from build123d import *

# Parameters (mm, degrees)
F0_W      = 31
F0_H      = 41
F1_DEPTH  = 12
F2_T      = -2
F3_R      = 1.5
F4_DEPTH  = 25
F6_DEPTH  = 25
F7_W      = 14.291796
F7_H      = 4
F8_DEPTH  = 1
F9_W      = 12
F9_H      = 2
F10_DEPTH = 11
F11_W     = 23
F11_H     = 30
F12_DEPTH = 12
F13_W     = 19
F13_H     = 28
F14_DEPTH = 7
F15_W     = 19
F15_H     = 4
F16_DEPTH = 4
F18_DEPTH = 25
F19_R     = 3.5
F20_DEPTH = 25
F21_W     = 27
F21_H     = 27
F22_DEPTH = 12
F23_W     = 27
F23_H     = 27
F23_W_2   = 15
F23_H_2   = 15
F24_DEPTH = 1
F25_W     = 10.156876
F25_H     = 2
F26_DEPTH = 10
F27_W     = 10
F27_H     = 2
F28_DEPTH = 7


with BuildPart() as f1:
    # F0 (on Top) → F1 (new body)
    with BuildSketch(Plane.XY):
        with Locations((15.5, 20.5)):
            Rectangle(F0_W, F0_H)
    extrude(amount=F1_DEPTH)

    # F2
    f2_openings = [f1.faces().sort_by_distance(p)[0] for p in [
        (15.5, 20.5, 12),
    ]]
    offset(amount=F2_T, openings=f2_openings)

    # F3 (on face) → F4 (cut)
    with BuildSketch(Plane.XY.offset(2)):
        with Locations((5, 36)):
            Circle(F3_R)
        with Locations((26, 36)):
            Circle(F3_R)
        with Locations((26, 5)):
            Circle(F3_R)
        with Locations((5, 5)):
            Circle(F3_R)
    extrude(amount=-F4_DEPTH, mode=Mode.SUBTRACT)

    # F5 (on face) → F6 (cut)
    with BuildSketch(Plane.XY.offset(2)):
        with BuildLine():
            ThreePointArc((25, 32.645898), (23.525126, 33.525126), (22.645898, 35))
            Line((22.645898, 35), (8.354102, 35))
            ThreePointArc((8.354102, 35), (7.474874, 33.525126), (6, 32.645898))
            Line((6, 32.645898), (6, 8.354102))
            ThreePointArc((6, 8.354102), (7.474874, 7.474874), (8.354102, 6))
            Line((8.354102, 6), (22.645898, 6))
            ThreePointArc((22.645898, 6), (23.525126, 7.474874), (25, 8.354102))
            Line((25, 8.354102), (25, 32.645898))
        make_face()
    extrude(amount=-F6_DEPTH, mode=Mode.SUBTRACT)

    # F7 (on face) → F8 (cut)
    with BuildSketch(Plane.XY.offset(2)):
        with Locations((15.5, 4)):
            Rectangle(F7_W, F7_H)
    extrude(amount=-F8_DEPTH, mode=Mode.SUBTRACT)

    # F9 (on face) → F10 (cut)
    with BuildSketch(Plane.XY.offset(12)):
        with Locations((15.5, 1)):
            Rectangle(F9_W, F9_H)
    extrude(amount=-F10_DEPTH, mode=Mode.SUBTRACT)

    # F11 (on face) → F12 (join)
    with BuildSketch(Plane(origin=(0, 0, 0), x_dir=(1, 0, 0), z_dir=(0, 0, -1))):
        with Locations((15.5, 15)):
            Rectangle(F11_W, F11_H)
    extrude(amount=-F12_DEPTH)

    # F13 (on face) → F14 (cut)
    with BuildSketch(Plane.XY.offset(12)):
        with Locations((15.5, -14)):
            Rectangle(F13_W, F13_H)
    extrude(amount=-F14_DEPTH, mode=Mode.SUBTRACT)

    # F15 (on face) → F16 (cut)
    with BuildSketch(Plane.XY.offset(5)):
        with Locations((15.5, -2)):
            Rectangle(F15_W, F15_H)
    extrude(amount=-F16_DEPTH, mode=Mode.SUBTRACT)

    # F17 (on face) → F18 (cut)
    with BuildSketch(Plane.XY.offset(5)):
        Polygon((25, -4), (21, -4), (10, -4), (10, -24), (21, -24), (21, -20), (25, -20), align=None)
    extrude(amount=-F18_DEPTH, mode=Mode.SUBTRACT)

    # F19 (on face) → F20 (cut)
    with BuildSketch(Plane.XZ.offset(-39)):
        with Locations((13.913386, 6.684771)):
            Circle(F19_R)
    extrude(amount=-F20_DEPTH, mode=Mode.SUBTRACT)

    # F21 (on face) → F22 (join)
    with BuildSketch(Plane.XY.offset(12)):
        Polygon((29, 41), (31, 41), (31, 113), (0, 113), (0, 41), (2, 41), (2, 82), (29, 82), align=None)
        with Locations((15.5, 97.5)):
            Rectangle(F21_W, F21_H, mode=Mode.SUBTRACT)
    extrude(amount=-F22_DEPTH)

    # F23 (on face) → F24 (join)
    with BuildSketch(Plane(origin=(0, 0, 0), x_dir=(1, 0, 0), z_dir=(0, 0, -1))):
        with Locations((15.5, -97.5)):
            Rectangle(F23_W, F23_H)
        with Locations((15.5, -97.5)):
            Rectangle(F23_W_2, F23_H_2, mode=Mode.SUBTRACT)
    extrude(amount=-F24_DEPTH)

    # F25 (on face) → F26 (cut)
    with BuildSketch(Plane.XY.offset(12)):
        with Locations((15.545943, 83)):
            Rectangle(F25_W, F25_H)
    extrude(amount=-F26_DEPTH, mode=Mode.SUBTRACT)

    # F27 (on face) → F28 (cut)
    with BuildSketch(Plane.XY.offset(12)):
        with Locations((15.5, -29)):
            Rectangle(F27_W, F27_H)
    extrude(amount=-F28_DEPTH, mode=Mode.SUBTRACT)


solid = f1.part
Source: CAD feature listing. Evaluate the final solid. Frame: model axes, mm. A direction names the side the tool comes from. Give positions to 0.01 mm unless a question says otherwise; leave off trailing zeros. Order: outer loops, then holes, each group sorted by start corner. A loop starts at its lowest first (then second) coordinate and runs counter-clockwise, first axis right, second up. Notation, with made-up numbers: (25.5, 78) -> (80.5, 78) arc R17 ccw to (80.5, 97) -> close; hole circle Ø7 at (67, 53.5). An arc over 180 degrees is marked (long way). Use a Markdown table: item, result.
1) Mould query, pull axis Y, two halves, no side actions, for faces 4 (the flat face through (15.3, -30, 4.6)), 5 (the cylindrical face through (6.386, 4.425, 1.014)), 6 (the flat face through (0, 57, 6)). Classes: +Y half, -Y half, draft (parallel to the pull), parting line (faces both ways), or undercut.
Answer list:
| item | result |
|---|---|
| face 4 | -Y half |
| face 5 | undercut |
| face 6 | draft |
2) Section query B-B, the plane y = 62. Return the cut outline in (x, z).
Answer list:
| item | result |
|---|---|
| outline | (0, 0) -> (2, 0) -> (2, 12) -> (0, 12) -> close; (29, 0) -> (31, 0) -> (31, 12) -> (29, 12) -> close |
3) Section query C-C, the plane y = 17. Return the cut outline in (x, z), then the cut area to 3 significant figures.
Answer list:
| item | result |
|---|---|
| outline | (0, 0) -> (6, 0) -> (6, 2) -> (2, 2) -> (2, 12) -> (0, 12) -> close; (25, 0) -> (31, 0) -> (31, 12) -> (29, 12) -> (29, 2) -> (25, 2) -> close |
| area | 64.0 mm² |
4) Contact query for flat-ended pins moving along their axis: P1, Ø4, axis at x = 5, y = 5, coming from the +Z side; P2, Ø2.5, axis at x = 26, y = 36, coming from the +Z side. Output: stop coordinate, or through.
Answer list:
| item | result |
|---|---|
| P1 | z = 2 |
| P2 | through |
5) Ray query, line 1 along Y through (x, z) = (5, 0.9); line 2 along Y through (x, z) = (10, 7.75); line 3 along Y through (x, z) = (8, 7). Return the intervals inside material, ascending. Write a range as [from, to].
Answer list:
| item | result |
|---|---|
| line 1 | [-30, 3.5], [6.5, 34.5], [37.5, 41], [82, 113] |
| line 2 | [-30, -28], [39, 41], [82, 84], [111, 113] |
| line 3 | [-30, -28], [0, 2], [39, 41], [82, 84], [111, 113] |
6) Section query A-A, the plane y = 98.5. Return the cut outline in (x, z), then the cut area to 3 significant figures.
Answer list:
| item | result |
|---|---|
| outline | (0, 0) -> (8, 0) -> (8, 1) -> (2, 1) -> (2, 12) -> (0, 12) -> close; (23, 0) -> (31, 0) -> (31, 12) -> (29, 12) -> (29, 1) -> (23, 1) -> close |
| area | 60.0 mm² |
7) Reachability of faces 1 (the flat face through (2, 97, 7)), 2 (the flat face through (29, 0, 6)), 3 (the cylindrical face through (23.54, 33.51, 1.01)) from +Z, -Z, +X, -X, +Y, -Y: full face, straight path, thin tool, end or side. Return the list, or none.
Answer list:
| item | result |
|---|---|
| face 1 | +Z |
| face 2 | +Z, -Z, +X, -Y |
| face 3 | +Z, -Z |
